from build123d import *

# Parameters (mm, degrees)
F0_W      = 600
F0_H      = 1060
F1_DEPTH  = 280
F2_T      = -25
F3_R      = 4
F4_DEPTH  = 8
F6_DEPTH  = 30
F9_DEPTH  = 50
F10_DEPTH = 50
F11_DEPTH = 50.001


with BuildPart() as f1:
    # F0 (on Top) → F1 (new body)
    with BuildSketch(Plane.XY):
        with Locations((300, -530)):
            Rectangle(F0_W, F0_H)
    extrude(amount=F1_DEPTH)

    # F2
    f2_openings = [f1.faces().sort_by_distance(p)[0] for p in [
        (300, -530, 0),
    ]]
    offset(amount=F2_T, openings=f2_openings)

    # F3 (on face) → F4 (cut)
    with BuildSketch(Plane(origin=(0, 0, 0), x_dir=(1, 0, 0), z_dir=(0, 0, -1))):
        with Locations((10, 1050)):
            Circle(F3_R)
        with Locations((10, 881)):
            Circle(F3_R)
        with Locations((179, 1050)):
            Circle(F3_R)
        with Locations((590, 1050)):
            Circle(F3_R)
        with Locations((421, 1050)):
            Circle(F3_R)
        with Locations((590, 881)):
            Circle(F3_R)
        with Locations((10, 179)):
            Circle(F3_R)
        with Locations((10, 10)):
            Circle(F3_R)
        with Locations((179, 10)):
            Circle(F3_R)
        with Locations((421, 10)):
            Circle(F3_R)
        with Locations((590, 10)):
            Circle(F3_R)
        with Locations((590, 179)):
            Circle(F3_R)
    extrude(amount=-F4_DEPTH, mode=Mode.SUBTRACT)

    # F5 (on face) → F6 (join)
    with BuildSketch(Plane(origin=(0, 0, 255), x_dir=(1, 0, 0), z_dir=(0, 0, -1))):
        Polygon((115, 1035), (25, 1035), (25, 945), align=None)
        Polygon((485, 1035), (575, 945), (575, 1035), align=None)
        Polygon((115, 25), (25, 115), (25, 25), align=None)
        Polygon((575, 25), (575, 115), (485, 25), align=None)
    extrude(amount=F6_DEPTH)

    # F8 (on face) → F9 (join)
    with BuildSketch(Plane(origin=(0, 0, 0), x_dir=(1, 0, 0), z_dir=(0, 0, -1))):
        Polygon((202, 1058), (2, 1058), (2, 1018.136144), (2, 858), (14.5, 858), (27, 878.238261), (27, 990.695417), (66.770039, 1033), (182.782859, 1033), (202, 1045.5), align=None)
        Polygon((533.229961, 1033), (573, 990.695417), (573, 878.238261), (585.5, 858), (598, 858), (598, 1058), (398, 1058), (398, 1045.5), (417.217141, 1033), align=None)
        Polygon((14.5, 202), (2, 202), (2, 2), (202, 2), (202, 14.5), (182.782859, 27), (66.770039, 27), (27, 69.304583), (27, 181.761739), align=None)
        Polygon((533.229961, 27), (417.217141, 27), (398, 14.5), (398, 2), (598, 2), (598, 202), (585.5, 202), (573, 181.761739), (573, 69.304583), align=None)
    extrude(amount=F9_DEPTH)

    # F8 (on face) → F10 (join)
    with BuildSketch(Plane(origin=(0, 0, 0), x_dir=(1, 0, 0), z_dir=(0, 0, -1))):
        Polygon((202, 1058), (2, 1058), (2, 1018.136144), (2, 858), (14.5, 858), (27, 878.238261), (27, 990.695417), (66.770039, 1033), (182.782859, 1033), (202, 1045.5), align=None)
        Polygon((533.229961, 1033), (573, 990.695417), (573, 878.238261), (585.5, 858), (598, 858), (598, 1058), (398, 1058), (398, 1045.5), (417.217141, 1033), align=None)
        Polygon((14.5, 202), (2, 202), (2, 2), (202, 2), (202, 14.5), (182.782859, 27), (66.770039, 27), (27, 69.304583), (27, 181.761739), align=None)
        Polygon((533.229961, 27), (417.217141, 27), (398, 14.5), (398, 2), (598, 2), (598, 202), (585.5, 202), (573, 181.761739), (573, 69.304583), align=None)
    extrude(amount=F10_DEPTH)

    # F3 (on face) → F11 (cut, through all)
    with BuildSketch(Plane(origin=(0, 0, 0), x_dir=(1, 0, 0), z_dir=(0, 0, -1))):
        with Locations((10, 1050)):
            Circle(F3_R)
        with Locations((10, 881)):
            Circle(F3_R)
        with Locations((179, 1050)):
            Circle(F3_R)
        with Locations((590, 1050)):
            Circle(F3_R)
        with Locations((421, 1050)):
            Circle(F3_R)
        with Locations((590, 881)):
            Circle(F3_R)
        with Locations((10, 179)):
            Circle(F3_R)
        with Locations((10, 10)):
            Circle(F3_R)
        with Locations((179, 10)):
            Circle(F3_R)
        with Locations((421, 10)):
            Circle(F3_R)
        with Locations((590, 10)):
            Circle(F3_R)
        with Locations((590, 179)):
            Circle(F3_R)
    extrude(amount=F11_DEPTH, mode=Mode.SUBTRACT)


solid = f1.part
Read the model definition and answer for the solid it produces. Units are mm, in the model's axes. A direction names the side the tool comes from. Give positions to 0.01 mm unless a question says otherwise; leave off trailing zeros. Write each loop counter-clockwise with the first axis right and the second up, starting at its lowest first coordinate (ties: lowest second). Pieces come first, ordered by that corner, then holes. Notation, with made-up numbers: (79.25, 7.5) -> (112.25, 7.5) arc R12 ccw to (112.25, 18.5) -> close; hole circle Ø11 at (37, 26.25). An arc over 180 degrees is marked (long way). Answer as a JSON object with one key per item and string values. Group by question number.
1) Find section C-C (y = -426). Write down the section's boundary in (x, z).
2) Consider L1, parallel to Y at x = 10, z = -6.5; L2, parallel to Y at x = 421, z = -28; L3, parallel to Y at x = 297, z = 171. Determine where each line is inside the solid, lowest interval first. Write a range as from..to.
3) A tool of negligible diameter and unlimited length cuts with its end or side. For faces 4 (the flat face through (50, -43, -50)), 5 (the flat face through (40, -1021, 0)), 6 (the flat face through (497, -2, -25)), 7 (the flat face through (126, -27, -25)), from which of +Z, -Z, +X, -X, +Y, -Y can it reach the whole face along a straight path? Write none if from no direction.
4) Find section D-D (y = -141.5). Write down the section's boundary in (x, z), and give its area (4 significant figures).
5) Each of these flat-tipped pins is pushed along its axis until it touches: P1, Ø6, axis at x = 331.5, y = -464, coming from the -Z side; P2, Ø15, axis at x = 465.5, z = -27.5, coming from the +Y side; P3, Ø15, axis at y = -973.5, z = -17.5, coming from the -X side. Where does it stop, or does it pass through?
6) The mould has two halves that part along Y. Classify faces 1 (the flat face through (598, -101, -25)), 2 (the flat face through (103, -1058, -25)), 3 (the flat face through (560, -1021, 0)): +Y half, -Y half, draft (parallel to the pull), parting line (faces both ways), or undercut.
7) Find section B-B (x = 442.5). Write down the section's boundary in (y, z), and give its area (4 significant figures).
8) Find section A-A (z = 60.5). Write down the section's boundary in (x, y), and give its area (3 significant figures).
Values follow:
{
 "1": {"outline": "(0, 0) -> (25, 0) -> (25, 255) -> (575, 255) -> (575, 0) -> (600, 0) -> (600, 280) -> (0, 280) -> close"},
 "2": {"L1": "y = -1058..-1054, -1046..-885, -877..-858, -202..-183, -175..-14, -6..-2", "L2": "y = -1058..-1054, -1046..-1033, -27..-14, -6..-2", "L3": "y = -1060..-1035, -25..0"},
 "3": {"face 4": "-Z, +X, -X, +Y, -Y", "face 5": "none", "face 6": "-Z, +X, -X, +Y", "face 7": "-Z"},
 "4": {"outline": "(0, 0) -> (2, 0) -> (2, -50) -> (27, -50) -> (27, 0) -> (25, 0) -> (25, 255) -> (575, 255) -> (575, 0) -> (573, 0) -> (573, -50) -> (598, -50) -> (598, 0) -> (600, 0) -> (600, 280) -> (0, 280) -> close", "area": "30,250 mm2"},
 "5": {"P1": "stops at z = 255", "P2": "stops at y = -2", "P3": "stops at x = 2"},
 "6": {"face 1": "draft", "face 2": "-Y half", "face 3": "undercut"},
 "7": {"outline": "(-1060, 0) -> (-1058, 0) -> (-1058, -50) -> (-1033, -50) -> (-1033, 0) -> (-1035, 0) -> (-1035, 255) -> (-25, 255) -> (-25, 0) -> (-27, 0) -> (-27, -50) -> (-2, -50) -> (-2, 0) -> (0, 0) -> (0, 280) -> (-1060, 280) -> close", "area": "41,750 mm2"},
 "8": {"outline": "(0, -1060) -> (600, -1060) -> (600, 0) -> (0, 0) -> close; hole (25, -1035) -> (575, -1035) -> (575, -25) -> (25, -25) -> close", "area": "80,500 mm2"}
}
